Geometry check sheet. Reference: the model listing, model coordinates, mm. Face numbers are marked on the shaded views. A direction names the side the tool comes from. Give positions to 0.01 mm unless a question says otherwise; leave off trailing zeros. Loops run counter-clockwise (first coordinate to the right, second up) from the corner with the lowest first, then second, coordinate; pieces in that order, holes last. Notation, with made-up numbers: (49.5, -12.5) -> (83.5, -12.5) arc R26 cw to (83.5, 4.5) -> close; hole circle Ø3 at (37.25, 51). An arc over 180 degrees is marked (long way). Write item = value, one per line.
Autodesk Inventor part; units mm, degrees
ref_plane "YZ Plane" through (0, 0, 0) normal (1, 0, 0) x (0, 1, 0)
ref_plane "XZ Plane" through (0, 0, 0) normal (0, 1, 0) x (-1, 0, 0)
ref_plane "XY Plane" through (0, 0, 0) normal (0, 0, 1) x (1, 0, 0)
sketch "Sketch1" plane through (0, 0, 0) normal (0, 0, 1) x (1, 0, 0)
  line L0 (-21.25, 21.25) -> (21.25, 21.25)
  line L1 (21.25, 21.25) -> (21.25, -21.25)
  line L2 (21.25, -21.25) -> (-21.25, -21.25)
  line L3 (-21.25, -21.25) -> (-21.25, 21.25)
  line L4 (-35, -35) -> (35, -35)
  line L5 (35, -35) -> (35, 35)
  line L6 (35, 35) -> (-35, 35)
  line L7 (-35, 35) -> (-35, -35)
  line L8 (-9, 35) -> (-9, 21.25)
  line L9 (9, 21.25) -> (9, 35)
  point P0 (0, 0)
  point P1 (-21.25, 0)
  point P2 (0, 21.25)
  point P3 (-35, 0)
  point P4 (0, 35)
  dimension "d0" = 42.5
  dimension "d1" = 9
  dimension "d3" = 70
  dimension "d17" = 18
extrude "Extrusion1" add sketch "Sketch1" along normal blind 45 contours L3 L2 L1 L0 L9 L6 L5 L4 L7 L8
sketch "Sketch4" plane through (0, 0, 0) normal (1, 0, 0) x (0, 1, 0)
  line L0 (-0.9, -15.9) -> (-21, -15.9)
  line L1 (-21, -15.9) -> (-21, -36)
  line L2 (-21, -36) -> (-0.9, -36)
  line L3 (-0.9, -36) -> (-0.9, -15.9)
  line L4 (-35, 0) -> (-35, 45)
  line L5 (7, -6) -> (7, -44)
  line L6 (7, -44) -> (-35, -44)
  line L7 (-35, -44) -> (-35, 0)
  line L8 (7, -6) -> (-10, -6)
  line L9 (-10, -6) -> (-10, 0)
  line L10 (-10, 0) -> (-35, 0)
  point P0 (0, 0)
  dimension "d18" = 20.1
  dimension "d20" = 14
  dimension "d21" = 42
  dimension "d22" = 38
  dimension "d30" = 8
  dimension "d31" = 6
  dimension "d32" = 25
extrude "Extrusion5" add sketch "Sketch4" along normal mid plane 120
sketch "Sketch5" plane through (60, 7, -44) normal (0, 0, -1) x (-1, 0, 0)
  circle A0 centre (15, -17.95) radius 2.15
  circle A1 centre (105, -17.95) radius 2.15
  line L0 (120, -7.9) -> (120, -7.9)
  line L1 (120, 0) -> (120, -42)
  line L2 (0, -42) -> (0, 0)
  line L3 (120, -28) -> (120, -7.9)
  point P0 (60, -7)
  point P1 (120, -21)
  point P2 (120, -17.95)
  dimension "d27" = 4.3
  dimension "d58" = 15
  dimension "d59" = 15
extrude "Extrusion6" cut sketch "Sketch5" against normal blind 18
sketch "Sketch6" plane through (9, 35, 0) normal (0, 1, 0) x (1, 0, 0)
  line L0 (26, 0) -> (0, 0)
  line L1 (0, 0) -> (8, 0)
  line L2 (8, 0) -> (8, -45)
  line L3 (8, -45) -> (0, -45)
  line L4 (0, -45) -> (0, 0)
  line L5 (-18, 0) -> (-18, -45)
  line L6 (-18, 0) -> (-26, 0)
  line L7 (-26, 0) -> (-26, -45)
  line L8 (-26, -45) -> (-18, -45)
  line L9 (-18, -45) -> (-18, 0)
  line L10 (26, -45) -> (0, -45)
  point P0 (-9, 0)
  dimension "d39" = 8
extrude "Extrusion7" add sketch "Sketch6" along normal blind 10
sketch "Sketch7" plane through (17, 35, 45) normal (1, 0, 0) x (0, 0, -1)
  circle A0 centre (12.5, 5) radius 1.6
  circle A1 centre (32.5, 5) radius 1.6
  line L0 (45, 10) -> (0, 10)
  point P0 (45, -35)
  point P1 (22.5, 10)
  dimension "d42" = 20
  dimension "d43" = 10
  dimension "d44" = 5
  dimension "d45" = 3.2
extrude "Extrusion8" cut sketch "Sketch7" against normal through all
sketch "Sketch8" plane through (-17, 35, 0) normal (-1, 0, 0) x (0, 0, 1)
  circle A0 centre (12.5, 5) radius 1.6
  circle A1 centre (32.5, 5) radius 1.6
  circle A2 centre (12.5, 5) radius 2.1
  circle A3 centre (32.5, 5) radius 2.1
  point P0 (0, -35)
  dimension "d48" = 4.2
extrude "Extrusion9" cut sketch "Sketch8" against normal blind 6
chamfer "Chamfer1" distance 25 angle 45 1 edges at (-35, -22.5, 0)
chamfer "Chamfer2" distance 35 distance2 25 1 edges at (35, -22.5, 0) measured on face at (35, -3.3333, 30)
chamfer "Chamfer3" distance 12.25 angle 45 2 edges at (-9, 21.25, 22.5) (9, 21.25, 22.5)
equation "\"d59\" = d58"
properties part number "Motorhalterig"
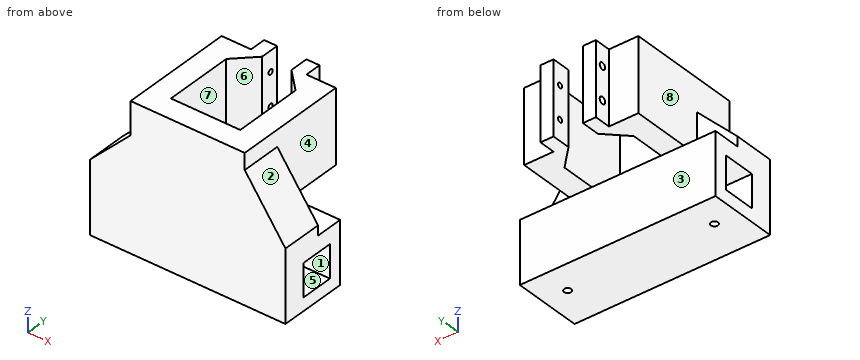
Item 1: Draft check along Y on the marked faces 1, 2 and 3. Enter one of: +Y half, -Y half, draft (parallel to the pull), parting line (faces both ways), or undercut.
Answer:
face_1 = undercut
face_2 = draft
face_3 = +Y half
Item 2: Section check C-C, the plane y = 40. Give the number of separate pieces and of enclosed holes in the cut face, plus the area to 3 significant figures.
Answer:
separate_pieces = 6
enclosed_holes = 0
area = 606 mm^2
Item 3: Tool access check on the marked faces 4, 5, 6, 7 and 8. Record the directions out of +Z, -Z, +X, -X, +Y, -Y that give a thin tool (end or side, any length) a straight path to the whole face; none if there is none.
Answer:
face_4 = +Z, +X, +Y
face_5 = +X, -X
face_6 = +Z, -Z
face_7 = +Z
face_8 = +Z, -X, +Y
Item 4: Section check D-D, the plane x = 37. Record the cut outline in (y, z).
Answer:
outline = (-35, -44) -> (7, -44) -> (7, -6) -> (-10, -6) -> (-10, 32.2) -> (-35, 32.2) -> close; hole (-21, -36) -> (-0.9, -36) -> (-0.9, -15.9) -> (-21, -15.9) -> close
Item 5: Thickness scan on L1, parallel to Y at x = 40.5, z = -29; L2, parallel to Y at x = -13.7, z = 12.5; L3, parallel to Z at x = 12, y = 33. Record the ranges inside material, lowest first. Write a range as [from, to].
Answer:
L1 = [-35, -21], [-0.9, 7]
L2 = [-35, -21.25], [28.8, 37.9], [42.1, 45]
L3 = [0, 45]
Item 6: Section check A-A, the plane y = 5. Record the cut outline in (x, z).
Answer:
outline = (-60, -44) -> (60, -44) -> (60, -6) -> (-60, -6) -> close; (-35, 0) -> (-21.25, 0) -> (-21.25, 45) -> (-35, 45) -> close; (21.25, 0) -> (35, 0) -> (35, 45) -> (21.25, 45) -> close
Item 7: Gauge pin test, flat ends, axial feed: pin 1 (3.5 mm diameter, centred on y = 40, z = 15, fed in from -X); pin 2 (1.5 mm diameter, centred on x = -37, z = 1.5, fed in from +Y); pin 3 (3.5 mm diameter, centred on y = 40, z = 32.5, fed in from +X); pin 4 (6 mm diameter, centred on x = 19.5, y = -13, fed in from +Z). Record the tip position at first contact, or that the pin passes through.
Answer:
pin_1 = -17
pin_2 = -10
pin_3 = 17
pin_4 = 45
Item 8: Section check B-B, the plane x = -13.5. Record the cut outline in (y, z).
Answer:
outline = (-35, -44) -> (7, -44) -> (7, -6) -> (-10, -6) -> (-10, 0) -> (-21.25, 0) -> (-21.25, 45) -> (-35, 45) -> close; (29, 0) -> (45, 0) -> (45, 45) -> (29, 45) -> close; hole (-21, -36) -> (-0.9, -36) -> (-0.9, -15.9) -> (-21, -15.9) -> close; hole circle Ø4.2 at (40, 12.5); hole circle Ø4.2 at (40, 32.5)
